from build123d import *

# Parameters (mm, degrees)
SKETCH1_W           = 106.1212
SKETCH1_H           = 120.8024
BOSS_EXTRUDE1_DEPTH = 5.7912
CAVITY2_START       = -53.0606
CAVITY2_OUTLINE_W   = 5.7912
CAVITY2_OUTLINE_H   = 5.7912
CAVITY2_DEPTH       = 35.373733333
CAVITY2_START_2     = 17.686866667
CAVITY2_2_OUTLINE_W = 5.7912
CAVITY2_2_OUTLINE_H = 5.7912
CAVITY2_2_DEPTH     = 35.373733333
SKETCH6_W           = 33.443333333
SKETCH6_H           = 5.7912
CUT_EXTRUDE4_DEPTH  = 81.605646398
SKETCH4_W           = 2.0828
SKETCH4_H           = 6.1722
CUT_EXTRUDE5_DEPTH  = 81.605646398
CUT_EXTRUDE6_DEPTH  = 81.605646398
SKETCH2_W           = 5.7912
SKETCH2_H           = 40.267466666
CUT_EXTRUDE7_DEPTH  = 81.605646398
SKETCH7_R           = 1.615828467
SKETCH7_R_2         = 1.628881449
SKETCH7_R_3         = 1.612957286
SKETCH7_R_4         = 1.6
CUT_EXTRUDE8_DEPTH  = 81.605646398


# Read off the part's stored shape, not the designer's step: Cavity2
with BuildPart() as part:
    # Sketch1 → Boss-Extrude1 (new body)
    with BuildSketch(Plane.XY):
        Rectangle(SKETCH1_W, SKETCH1_H)
    extrude(amount=BOSS_EXTRUDE1_DEPTH)

    # Cavity2 outline → Cavity2 (cut)
    with BuildSketch(Plane.YZ.offset(CAVITY2_START)):
        with Locations((-57.5056, 2.8956)):
            Rectangle(CAVITY2_OUTLINE_W, CAVITY2_OUTLINE_H)
    extrude(amount=CAVITY2_DEPTH, mode=Mode.SUBTRACT)

    # Cavity2 2 outline → Cavity2 2 (cut)
    with BuildSketch(Plane.YZ.offset(CAVITY2_START_2)):
        with Locations((-57.5056, 2.8956)):
            Rectangle(CAVITY2_2_OUTLINE_W, CAVITY2_2_OUTLINE_H)
    extrude(amount=CAVITY2_2_DEPTH, mode=Mode.SUBTRACT)

    # Sketch6 → Cut-Extrude4 (cut, through all)
    with BuildSketch(Plane(origin=(0, 0, 0), x_dir=(-1, 0, 0), z_dir=(0, 0, -1))):
        with Locations((-36.338933334, 57.5056)):
            Rectangle(SKETCH6_W, SKETCH6_H)
        with Locations((36.338933334, 57.5056)):
            Rectangle(SKETCH6_W, SKETCH6_H)
    extrude(amount=-CUT_EXTRUDE4_DEPTH, mode=Mode.SUBTRACT)

    # Sketch4 → Cut-Extrude5 (cut, through all)
    with BuildSketch(Plane(origin=(0, 0, 0), x_dir=(-1, 0, 0), z_dir=(0, 0, -1))):
        with Locations((-43.307, 0)):
            Rectangle(SKETCH4_W, SKETCH4_H)
    extrude(amount=-CUT_EXTRUDE5_DEPTH, mode=Mode.SUBTRACT)

    # Sketch3 → Cut-Extrude6 (cut, through all)
    with BuildSketch(Plane(origin=(0, 0, 0), x_dir=(-1, 0, 0), z_dir=(0, 0, -1))):
        Polygon((-50.0888, 1.30175), (-50.0888, -1.30175), (-36.5252, -1.30175), (-36.322002291, 1.29380831), align=None)
    extrude(amount=-CUT_EXTRUDE6_DEPTH, mode=Mode.SUBTRACT)

    # Sketch2 → Cut-Extrude7 (cut, through all)
    with BuildSketch(Plane(origin=(0, 0, 0), x_dir=(-1, 0, 0), z_dir=(0, 0, -1))):
        with Locations((-50.165, 0)):
            Rectangle(SKETCH2_W, SKETCH2_H)
        with Locations((50.165, 0)):
            Rectangle(SKETCH2_W, SKETCH2_H)
    extrude(amount=-CUT_EXTRUDE7_DEPTH, mode=Mode.SUBTRACT)

    # Sketch7 → Cut-Extrude8 (cut, through all)
    with BuildSketch(Plane.XY.offset(5.7912)):
        with Locations((5.9544, -46.06)):
            Circle(SKETCH7_R)
        with Locations((-27.0456, 6.34)):
            Circle(SKETCH7_R_2)
        with Locations((-21.9456, -46.06)):
            Circle(SKETCH7_R_3)
        with Locations((21.2544, 4.74)):
            Circle(SKETCH7_R_4)
    extrude(amount=-CUT_EXTRUDE8_DEPTH, mode=Mode.SUBTRACT)


solid = part.part
Here's how the part is built. I have some questions about the finished solid (model axes, mm). A direction names the side the tool comes from. Give positions to 0.01 mm unless a question says otherwise; leave off trailing zeros. Order: outer loops, then holes, each group sorted by start corner. A loop starts at its lowest first (then second) coordinate and runs counter-clockwise, first axis right, second up. Notation, with made-up numbers: (13.5, -1.75) -> (62.5, -1.75) arc R23 ccw to (62.5, 31.25) -> close; hole circle Ø11 at (28, -38.5). An arc over 180 degrees is marked (long way). Use a Markdown table: item, result. Add a question column.
Item 1: Imagine slicing it at C-C on z = 4.25. Give the number of separate pieces and of enclosed holes in the cut face, plus the area to 3 significant figures.
Item 2: Imagine slicing it at D-D on y = -7. Please give me the cut outline in (x, z).
Item 3: Will these pins go through, and if not, where does the flat tip stop? pin 1 (3 mm diameter, centred on x = -49.5, z = 2, fed in from -Y); pin 2 (0.9 mm diameter, centred on y = 2, z = 3, fed in from -X); pin 3 (3 mm diameter, centred on x = 46, z = 2.5, fed in from +Y); pin 4 (4 mm diameter, centred on x = -21.95, y = -46.06, fed in from +Z).
Item 4: Imagine slicing it at A-A on y = -46.06. Please give me the cut outline in (x, z), plus the area to 3 significant figures.
Item 5: Imagine slicing it at B-B on x = -42. Please give me the cut outline in (y, z).
Item 6: I need wall thicknesses on line 1 (Y direction, x = 41, z = 1.15); line 2 (X direction, y = 5, z = 3.85); line 3 (X direction, y = 6.5, z = 3.55). Which ranges of each line are inside material? Lowest first, please.
Item 7: If we mould it in two halves opening along Y, with no side actions, what happens to faces 4 (the face through (-17.687, -58, 3)), 5 (the face through (37, 54.61, 3)), 6 (the face through (5.74, -44.46, 2.94))? For each: pulls with the +Y half, pulls with the -Y half, needs draft (parallel to the pull), parting line crosses it, or undercut.
Item 8: For faces 1 (the face through (50, 20.134, 3)), 2 (the face through (17.687, -58, 3)), 3 (the face through (-47.269, 0, 3)), which set-ups out of +Z, -Z, +X, -X, +Y, -Y let a thin tool reach every point of the face, with its end or its side?
Data:
| question | item | result |
|---|---|---|
| 1 | separate pieces | 1 |
| 1 | enclosed holes | 4 |
| 1 | area | 11,500 mm² |
| 2 | outline | (-47.27, 0) -> (47.27, 0) -> (47.27, 5.79) -> (-47.27, 5.79) -> close |
| 3 | pin 1 | stops at y = -54.61 |
| 3 | pin 2 | stops at x = -47.27 |
| 3 | pin 3 | stops at y = 54.61 |
| 3 | pin 4 | stops at z = 5.79 |
| 4 | outline | (-53.06, 0) -> (-23.56, 0) -> (-23.56, 5.79) -> (-53.06, 5.79) -> close; (-20.33, 0) -> (4.34, 0) -> (4.34, 5.79) -> (-20.33, 5.79) -> close; (7.57, 0) -> (53.06, 0) -> (53.06, 5.79) -> (7.57, 5.79) -> close |
| 4 | area | 577 mm² |
| 5 | outline | (-54.61, 0) -> (54.61, 0) -> (54.61, 5.79) -> (-54.61, 5.79) -> close |
| 6 | line 1 | y = -54.61 to -1.3, 1.3 to 54.61 |
| 6 | line 2 | x = -47.27 to -27.97, -26.12 to 19.68, 22.83 to 47.27 |
| 6 | line 3 | x = -47.27 to -28.67, -25.42 to 47.27 |
| 7 | face 4 | needs draft |
| 7 | face 5 | pulls with the +Y half |
| 7 | face 6 | undercut |
| 8 | face 1 | +Z, -Z, +X |
| 8 | face 2 | +Z, -Z, +X, -Y |
| 8 | face 3 | +Z, -Z, -X |
